The model under review builds one solid part; all positions refer to its coordinate system, in mm. Coordinates: 2 decimals unless noted, no trailing zeros. Order: outer loops, then holes, each group sorted by start corner. A loop starts at its lowest first (then second) coordinate and runs counter-clockwise, first axis right, second up. Notation, with made-up numbers: M -25,-36.75 L 22,-36.75 A24 ccw 22,-6.75 Z; hole C 56.25,39.25 d6. An arc over 180 degrees is marked long. Answer as CSV lines item,"result". Start each with the question number.
Q1. Consider section A-A on x = 138. Write out the cut boundary in (y, z), and give its area (3 significant figures).
Q2. Consider section B-B on z = 20. Write out the cut boundary in (x, y), and give its area (3 significant figures).
Q3. Consider section C-C on y = 0.2. Write out the cut boundary in (x, z).
Q4. Wall thickness on L1, parallel to X at y = 0.75, z = -121.5; L2, parallel to Z at x = 72, y = 0.1; L3, parallel to X at y = 0.6, z = -19: over which ranges is each line inside the solid? List them lowest first. Write a range as [from, to].
Autodesk Inventor part; units mm, degrees
ref_plane "YZ Plane" through (0, 0, 0) normal (1, 0, 0) x (0, 1, 0)
ref_plane "XZ Plane" through (0, 0, 0) normal (0, 1, 0) x (-1, 0, 0)
ref_plane "XY Plane" through (0, 0, 0) normal (0, 0, 1) x (1, 0, 0)
sketch "Sketch1" plane through (0, 0, 0) normal (0, 1, 0) x (-1, 0, 0)
  line L0 (-168.1278, 70.4675) -> (181.8722, 70.4675)
  line L1 (181.8722, 70.4675) -> (181.8722, -319.5325)
  line L2 (181.8722, -319.5325) -> (-168.1278, -319.5325)
  line L3 (-168.1278, -319.5325) -> (-168.1278, 70.4675)
  circle A0 centre (6.8722, -124.5325) radius 160
  point P0 (0, 0)
  dimension "d0" = 350
  dimension "d1" = 390
  dimension "d2" = 320
extrude "Extrusion1" add sketch "Sketch1" along normal blind 0.8
properties part number "side350x390_hull"
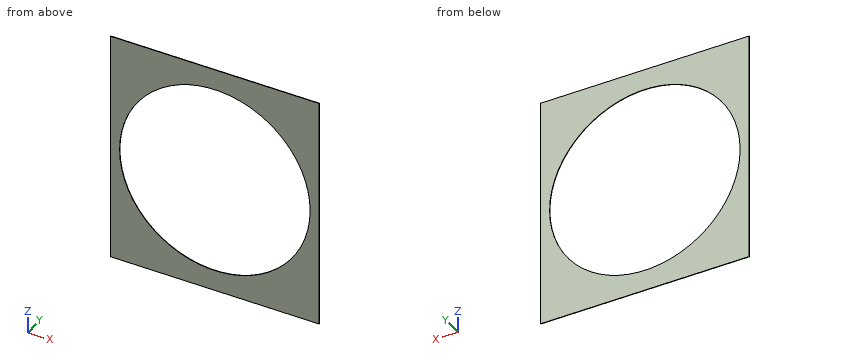
Evaluation:
1,outline,"M 0,-319.53 L 0.8,-319.53 L 0.8,-192.44 L 0,-192.44 Z; M 0,-56.62 L 0.8,-56.62 L 0.8,70.47 L 0,70.47 Z"
1,area,"203 mm²"
2,outline,"M -181.87,0 L -75.5,0 L -75.5,0.8 L -181.87,0.8 Z; M 61.76,0 L 168.13,0 L 168.13,0.8 L 61.76,0.8 Z"
2,area,"170 mm²"
3,outline,"M -181.87,-319.53 L 168.13,-319.53 L 168.13,70.47 L -181.87,70.47 Z; hole C -6.87,-124.53 d320"
4,L1,"x = [-181.87, -166.84], [153.1, 168.13]"
4,L2,"z = [-319.53, -263.74], [14.68, 70.47]"
4,L3,"x = [-181.87, -127.13], [113.39, 168.13]"
